from build123d import *

# Parameters (mm, degrees)
SKETCH1_R            = 3.96875
BOSS_EXTRUDE2_DEPTH  = 40.64
SKETCH7_W            = 321.437634852
SKETCH7_H            = 153.081921076
CUT_EXTRUDE3_DEPTH   = 33.02
EXTRUDE_THIN1_DEPTH  = 10
SKETCH14_R           = 1.950000064
CUT_EXTRUDE6_DEPTH   = 20
BOSS_EXTRUDE4_DEPTH  = 5
MIRROR5_COPY_1_DEPTH = 5
FILLET3_R            = 2.54
SKETCH20_W           = 13.97
SKETCH20_H           = 5.08
BOSS_EXTRUDE5_DEPTH  = 10
FILLET7_SIZE         = 3.81
FILLET7_SIZE_2       = 5.08
FILLET6_SIZE         = 3.81
FILLET6_SIZE_2       = 5.08
CUT_EXTRUDE10_START  = -5
SKETCH19_W           = 7.62
SKETCH19_H           = 10.16
CUT_EXTRUDE10_DEPTH  = 6.27
MIRROR6_OUTLINE_W    = 7.62
MIRROR6_OUTLINE_H    = 5
MIRROR6_DEPTH        = 10
MIRROR6_2_DEPTH      = 10
SKETCH21_W           = 77.087164644
SKETCH21_H           = 69.073945867
CUT_EXTRUDE11_DEPTH  = 210.74909516
SKETCH23_R           = 5.08
CUT_EXTRUDE12_DEPTH  = 255.54404949
SKETCH22_R           = 4.953
CUT_EXTRUDE13_DEPTH  = 255.54404949
CUT_EXTRUDE14_START  = 19.05
SKETCH24_W           = 240.575030827
SKETCH24_H           = 80.300707095
CUT_EXTRUDE14_DEPTH  = 235.389112867
SKETCH25_R           = 25.4
CUT_EXTRUDE15_DEPTH  = 5
FILLET10_R           = 1.905


# Read off the part's stored shape, not the designer's step: Mirror6
with BuildPart() as part:
    # Sketch1 → Boss-Extrude2 (new body)
    with BuildSketch(Plane(origin=(0, 0, 0), x_dir=(1, 0, 0), z_dir=(0, 1, 0))):
        with BuildLine():
            Line((-96.52, 178.942765331), (-55.88, 178.942765331))
            ThreePointArc((-55.88, 178.942765331), (-52.287897552, 177.454867779), (-50.8, 173.862765331))
            Line((-50.8, 173.862765331), (-50.8, 154.610881096))
            ThreePointArc((-50.8, 154.610881096), (-50.750979429, 153.906859803), (-50.604863787, 153.216425724))
            Line((-50.604863787, 153.216425724), (-23.277092285, 57.485544628))
            ThreePointArc((-23.277092285, 57.485544628), (-21.451849938, 54.824742099), (-18.392228498, 53.8))
            Line((-18.392228498, 53.8), (0, 53.8))
            Line((0, 53.8), (0, 0))
            Line((0, 0), (-40.91748188, 0))
            ThreePointArc((-40.91748188, 0), (-43.817717665, 0.909264766), (-45.679732106, 3.31156205))
            Line((-45.679732106, 3.31156205), (-101.282250226, 153.044327381))
            ThreePointArc((-101.282250226, 153.044327381), (-101.519931557, 153.914386555), (-101.6, 154.812765331))
            Line((-101.6, 154.812765331), (-101.6, 173.862765331))
            ThreePointArc((-101.6, 173.862765331), (-100.112102448, 177.454867779), (-96.52, 178.942765331))
        make_face()
        with Locations(Location((-88.9, 166.242765331, 0), (0, 0, 270))):
            Circle(SKETCH1_R, mode=Mode.SUBTRACT)
        with Locations(Location((-63.5, 166.242765331, 0), (0, 0, 270))):
            Circle(SKETCH1_R, mode=Mode.SUBTRACT)
    boss_extrude2 = extrude(amount=BOSS_EXTRUDE2_DEPTH)

    # Mirror1: Boss-Extrude2 across plane
    add(boss_extrude2.mirror(Plane(origin=(0, 40.64, -53.8), x_dir=(0, 0, 1), z_dir=(-1, 0, 0))))

    # Sketch7 → Cut-Extrude3 (cut)
    with BuildSketch(Plane(origin=(0, 40.64, 0), x_dir=(1, 0, 0), z_dir=(0, 1, 0))):
        with Locations((5.589227859, 76.540960538)):
            Rectangle(SKETCH7_W, SKETCH7_H)
    extrude(amount=-CUT_EXTRUDE3_DEPTH, mode=Mode.SUBTRACT)

    # Sketch9 → Extrude-Thin1 (add)
    with BuildSketch(Plane(origin=(0, 0, 0), x_dir=(1, 0, 0), z_dir=(0, 1, 0))):
        Polygon((-91.44, 173.942765331), (-91.44, 224.742765331), (-60.96, 224.742765331), (-60.96, 173.942765331), (-65.96, 173.942765331), (-65.96, 219.742765331), (-86.44, 219.742765331), (-86.44, 173.942765331), align=None)
    extrude_thin1 = extrude(amount=EXTRUDE_THIN1_DEPTH)

    # Sketch14 → Cut-Extrude6 (cut)
    with BuildSketch(Plane.XZ):
        with Locations(Location((-81.2, -174.942765331, 0), (0, 0, 270))):
            Circle(SKETCH14_R)
        with Locations(Location((-71.2, -174.942765331, 0), (0, 0, 270))):
            Circle(SKETCH14_R)
    cut_extrude6 = extrude(amount=-CUT_EXTRUDE6_DEPTH, mode=Mode.SUBTRACT)

    # Sketch18 → Boss-Extrude4 (add)
    with BuildSketch(Plane(origin=(-60.96, 10, -178.942765331), x_dir=(0, 0, 1), z_dir=(-1, 0, 0))):
        Polygon((-1.27, 0), (0, 1.524), (0, 0), align=None)
    boss_extrude4 = extrude(amount=BOSS_EXTRUDE4_DEPTH)

    # Mirror3: Boss-Extrude4 across plane
    add(boss_extrude4.mirror(Plane(origin=(-76.2, 0, 0), x_dir=(0, 0, 1), z_dir=(1, 0, 0))))

    # Mirror5: Extrude-Thin1, Cut-Extrude6, Boss-Extrude4 across plane
    add(extrude_thin1.mirror(Plane(origin=(0, 0, 0), x_dir=(0, 0, 1), z_dir=(1, 0, 0))))
    add(cut_extrude6.mirror(Plane(origin=(0, 0, 0), x_dir=(0, 0, 1), z_dir=(1, 0, 0))), mode=Mode.SUBTRACT)
    add(boss_extrude4.mirror(Plane(origin=(0, 0, 0), x_dir=(0, 0, 1), z_dir=(1, 0, 0))))

    # Mirror5 copy 1 sketch → Mirror5 copy 1 (add)
    with BuildSketch(Plane(origin=(91.44, 10, -178.942765331), x_dir=(0, 0, 1), z_dir=(-1, 0, 0))):
        Polygon((-1.27, 0), (0, 1.524), (0, 0), align=None)
    extrude(amount=MIRROR5_COPY_1_DEPTH)

    # Fillet3
    fillet3_edges = [part.edges().sort_by_distance(p)[0] for p in [
        (-91.44, 5, -224.742765331),
        (-60.96, 5, -224.742765331),
        (91.44, 5, -224.742765331),
        (60.96, 5, -224.742765331),
    ]]
    fillet(fillet3_edges, radius=FILLET3_R)

    # Sketch20 → Boss-Extrude5 (add)
    with BuildSketch(Plane(origin=(0, 0, 0), x_dir=(1, 0, 0), z_dir=(0, 1, 0))):
        with Locations((-76.2, 227.282765331)):
            Rectangle(SKETCH20_W, SKETCH20_H)
    extrude(amount=BOSS_EXTRUDE5_DEPTH)

    # Fillet7
    # an asymmetric fillet: 5.08, 3.81 mm, written as the material it takes off along each edge
    with BuildSketch(Plane(origin=(-83.185, -12.7, -229.822765331), x_dir=(0, 0, 1), z_dir=(0, 1, 0))) as fillet7_piece_1:
        with BuildLine():
            Bezier((FILLET7_SIZE, 0), (0, 0), (0, FILLET7_SIZE_2), weights=[1, 0.707106781, 1])
            Line((0, FILLET7_SIZE_2), (0, 0))
            Line((0, 0), (FILLET7_SIZE, 0))
        make_face()
    extrude(amount=35.4, mode=Mode.SUBTRACT)

    # Fillet6
    # an asymmetric fillet: 5.08, 3.81 mm, written as the material it takes off along each edge
    with BuildSketch(Plane(origin=(-69.215, -12.7, -229.822765331), x_dir=(0, 0, 1), z_dir=(0, 1, 0))) as fillet6_piece_1:
        with BuildLine():
            Bezier((FILLET6_SIZE, 0), (0, 0), (0, -FILLET6_SIZE_2), weights=[1, 0.707106781, 1])
            Line((0, -FILLET6_SIZE_2), (0, 0))
            Line((0, 0), (FILLET6_SIZE, 0))
        make_face()
    extrude(amount=35.4, mode=Mode.SUBTRACT)

    # Sketch19 → Cut-Extrude10 (cut)
    with BuildSketch(Plane(origin=(0, 0, -224.742765331), x_dir=(-1, 0, 0), z_dir=(0, 0, -1)).offset(CUT_EXTRUDE10_START)):
        with Locations((76.2, 4.92)):
            Rectangle(SKETCH19_W, SKETCH19_H)
    extrude(amount=CUT_EXTRUDE10_DEPTH, mode=Mode.SUBTRACT)

    # Mirror6 outline → Mirror6 (cut)
    with BuildSketch(Plane(origin=(0, 0, 0), x_dir=(1, 0, 0), z_dir=(0, 1, 0))):
        with Locations((76.2, 222.242765331)):
            Rectangle(MIRROR6_OUTLINE_W, MIRROR6_OUTLINE_H)
    extrude(amount=MIRROR6_DEPTH, mode=Mode.SUBTRACT)

    # Mirror6 2 outline → Mirror6 2 (add)
    with BuildSketch(Plane(origin=(0, 0, 0), x_dir=(1, 0, 0), z_dir=(0, 1, 0))):
        with BuildLine():
            add(Edge.make_bspline(
                [(78.105, 229.822765331), (83.185, 229.822765331), (83.185, 226.012765331)],
                knots=[0, 0, 0, 1, 1, 1], degree=2, weights=[1, 0.707106781, 1]))
            Line((78.105, 229.822765331), (74.295, 229.822765331))
            add(Edge.make_bspline(
                [(69.215, 226.012765331), (69.215, 229.822765331), (74.295, 229.822765331)],
                knots=[0, 0, 0, 1, 1, 1], degree=2, weights=[1, 0.707106781, 1]))
            Line((69.215, 226.012765331), (69.215, 224.742765331))
            Line((69.215, 224.742765331), (72.39, 224.742765331))
            Line((72.39, 224.742765331), (72.39, 226.012765331))
            Line((72.39, 226.012765331), (80.01, 226.012765331))
            Line((80.01, 226.012765331), (80.01, 224.742765331))
            Line((80.01, 224.742765331), (83.185, 224.742765331))
            Line((83.185, 224.742765331), (83.185, 226.012765331))
        make_face()
    extrude(amount=MIRROR6_2_DEPTH)

    # Sketch21 → Cut-Extrude11 (cut, through all)
    with BuildSketch(Plane(origin=(0, 0, -178.942765331), x_dir=(-1, 0, 0), z_dir=(0, 0, -1))):
        with Locations((78.752430528, 22.788762469)):
            Rectangle(SKETCH21_W, SKETCH21_H)
    extrude(amount=CUT_EXTRUDE11_DEPTH, mode=Mode.SUBTRACT)

    # Sketch23 → Cut-Extrude12 (cut, through all)
    with BuildSketch(Plane.XZ):
        with Locations((-67.31, -98.573931837)):
            Circle(SKETCH23_R)
        with Locations((-71.958522628, -103.222454465)):
            Circle(SKETCH23_R)
        with Locations((-60.96, -96.872454465)):
            Circle(SKETCH23_R)
        with Locations((-54.61, -98.573931837)):
            Circle(SKETCH23_R)
        with Locations((-49.961477372, -103.222454465)):
            Circle(SKETCH23_R)
    extrude(amount=-CUT_EXTRUDE12_DEPTH, mode=Mode.SUBTRACT)

    # Sketch22 → Cut-Extrude13 (cut, through all)
    with BuildSketch(Plane.XZ):
        with Locations(Location((-60.96, -109.572454465, 0), (0, 0, 270))):
            Circle(SKETCH22_R)
    extrude(amount=-CUT_EXTRUDE13_DEPTH, mode=Mode.SUBTRACT)

    # Sketch24 → Cut-Extrude14 (cut, through all)
    with BuildSketch(Plane(origin=(0, 7.62, 0), x_dir=(1, 0, 0), z_dir=(0, 1, 0)).offset(CUT_EXTRUDE14_START)):
        with Locations((-12.016343346, 155.193868331)):
            Rectangle(SKETCH24_W, SKETCH24_H)
    extrude(amount=CUT_EXTRUDE14_DEPTH, mode=Mode.SUBTRACT)

    # Sketch25 → Cut-Extrude15 (cut)
    with BuildSketch(Plane(origin=(0, 7.62, 0), x_dir=(1, 0, 0), z_dir=(0, 1, 0))):
        with Locations((0, 25.352)):
            Circle(SKETCH25_R)
    extrude(amount=-CUT_EXTRUDE15_DEPTH, mode=Mode.SUBTRACT)

    # Fillet10
    fillet10_edges = [part.edges().sort_by_distance(p)[0] for p in [
        (0, 2.62, 0),
        (-1.560799795, 5.12, 0),
        (1.560799795, 5.12, 0),
    ]]
    fillet(fillet10_edges, radius=FILLET10_R)


with BuildPart() as body_2:
    # Mirror16: mirrored copy
    add(part.part.mirror(Plane(origin=(119.38, 0, 0), x_dir=(0, 0, 1), z_dir=(1, 0, 0))))


solid = body_2.part
Geometry: final body of the model. Coordinates: model frame, mm. A direction names the side the tool comes from. Give positions to 0.01 mm unless a question says otherwise; leave off trailing zeros. Loops run counter-clockwise (first coordinate to the right, second up) from the corner with the lowest first, then second, coordinate; pieces in that order, holes last. Notation, with made-up numbers: M 87,56 L 96,56 A34 ccw 96,86 Z; hole C 26,-8.5 d1. An arc over 180 degrees is marked long. Put each result on its own line as item: value. Start each with the question number.
1) Cut plane A-A (z = -200.5). Output: boundary loops of the cut face in (x, y).
2) Ray query, line 1 along X through (y, z) = (22, -166); line 2 along Z through (x, y) = (175.5, 9.75); line 3 along Y through (x, z) = (221, -15.5). Return the intervals inside material, ascending.
3) Contact query for flat-ended pins moving along their axis: pin 1 (10 mm diameter, centred on x = 313.5, z = -128.5, fed in from +Y); pin 2 (4.5 mm diameter, centred on x = 173.5, y = 3.5, fed in from -Z); pin 3 (12.5 mm diameter, centred on y = 5.5, z = -197.5, fed in from +X). Output: stop coordinate, or through.
4) Pull-direction query (Z, two-part tool) for faces 5 (the flat face through (208, 0, -81)), 6 (the cylindrical face through (290.77, 3.76, -94.21)), 7 (the flat face through (239, 4, -53.8)), 8 (the flat face through (311.85, 3.76, -77.13)); classes: pulls with the +Z half, pulls with the -Z half, needs draft (parallel to the pull), parting line crosses it, or undercut.
5) Cut plane D-D (x = 208.5). Output: boundary loops of the cut face in (y, z), then the cut area to 3 significant figures.
6) Access query for faces 1 (the cylindrical face through (308.55, 3.76, -94.14)), 2 (the flat face through (177.8, 6, -200)), 3 (the flat face through (152, 10, -205)), 4 (the cylindrical face through (291.088, 13.148, -177.494)). Directions: +Z, -Z, +X, -X, +Y, -Y. A direction counts if a zero-diameter tool reaches every point of the face in a straight line with its end or side. Return the directions, or none.
7) Cut plane C-C (z = -74). Output: boundary loops of the cut face in (x, y).
8) Cut plane B-B (z = -19). Output: boundary loops of the cut face in (x, y).
Verdict:
1. outline: M 147.32,0 L 152.32,0 L 152.32,10 L 147.32,10 Z; M 172.8,0 L 177.8,0 L 177.8,10 L 172.8,10 Z
2. line 1: 137.16 to 145.9, 153.82 to 171.3, 179.22 to 187.96, 289.56 to 298.3, 306.22 to 323.7, 331.62 to 340.36
2. line 2: -224.73 to -170.2, -162.28 to -153.08
2. line 3: 0 to 2.62
3. pin 1: y = 7.62
3. pin 2: z = -224.74
3. pin 3: x = 177.8
4. face 5: needs draft
4. face 6: undercut
4. face 7: pulls with the -Z half
4. face 8: pulls with the +Z half
5. outline: M 0,-81.95 L 7.62,-81.95 L 7.62,0 L 0,0 Z
5. area: 624 mm2
6. face 1: +Y, -Y
6. face 2: -Z, +X, +Y, -Y
6. face 3: -Z, +X, -X, +Y
6. face 4: -Z, +Y, -Y
7. outline: M 166.83,0 L 210.77,0 L 210.77,7.62 L 166.83,7.62 Z; M 266.75,0 L 310.69,0 L 310.69,7.62 L 266.75,7.62 Z
8. outline: M 187.25,0 L 290.27,0 L 290.27,7.62 L 263.35,7.62 L 263.35,2.62 L 214.17,2.62 L 214.17,7.62 L 187.25,7.62 Z
